Could you check a few things on this model? Use its own coordinates, in mm. A direction names the side the tool comes from. Round coordinates to 2 decimals unless told otherwise and drop trailing zeros. Order: outer loops, then holes, each group sorted by start corner. A loop starts at its lowest first (then second) coordinate and runs counter-clockwise, first axis right, second up.
Solid Edge part; units mm, degrees
sketch "Sketch1" plane through (0, 0, 0) normal (0, 0, 1) x (1, 0, 0)
  circle A0 centre (0, 0) radius 10.5
extrude "Protrusion1" add sketch "Sketch1" along normal blind 2
sketch "Sketch2" plane through (0, 0, 2) normal (0, 0, 1) x (1, 0, 0)
  line L0 (-3.25, -3.25) -> (3.25, -3.25)
  line L1 (3.25, -3.25) -> (3.25, 3.25)
  line L2 (3.25, 3.25) -> (-3.25, 3.25)
  line L3 (-3.25, 3.25) -> (-3.25, -3.25)
extrude "Extrusionsausprägung_2" add sketch "Sketch2" along normal blind 6.5
chamfer "Fase_1" distance 1 angle 45 1 edges at (-10.5, 0, 2)
hole "Bohrung_1" at (0, 0, 0) direction (0, 0, 1) diameter 4 end through all
Q1. Imagine slicing it at A-A, the plane x = 0. Please give me the cut outline in (y, z).
Q2. Imagine slicing it at C-C, the plane z = 1.5. Please give me the cut outline in (x, y).
Q3. We'd pull the mould along X, two halves only. Please class faces 4 (the cylindrical face through (-2, 0, 4)), 5 (the flat face through (0, 3.25, 5)), 6 (the flat face through (-3.25, 0, 5)): released by +X, released by -X, zero draft, split by the parting line, or undercut.
Q4. For faces 1 (the flat face through (2.2, 0.1, 0)), 2 (the flat face through (3.25, 0, 5)), 3 (the flat face through (0, -3.25, 5)), which set-ups out of +Z, -Z, +X, -X, +Y, -Y let a thin tool reach every point of the face, with its end or its side?
Q5. Imagine slicing it at D-D, the plane z = 2.75. Please give me the cut outline in (x, y), then the cut area to 3 significant figures.
Q6. I need wall thicknesses on L1, parallel to X at y = 0, z = 4; L2, parallel to Z at x = -4, y = 5. Which ranges of each line are inside material? Lowest first, please.
Q7. For P1, Ø5, axis at x = -0.5, z = 6, coming from the -Y side; P2, Ø5, axis at x = 6, z = 1, coming from the +Y side; P3, Ø3, axis at y = -4, z = 2, coming from the -X side, each with a flat end and sliding along its axis, tell me the tip position at first contact or that it passes through.
Filled in:
1. outline: (-10.5, 0) - (-2, 0) - (-2, 8.5) - (-3.25, 8.5) - (-3.25, 2) - (-9.5, 2) - (-10.5, 1) - close; (2, 0) - (10.5, 0) - (10.5, 1) - (9.5, 2) - (3.25, 2) - (3.25, 8.5) - (2, 8.5) - close
2. outline: circle Ø20 at (0, 0); hole circle Ø4 at (0, 0)
3. face 4: undercut
3. face 5: zero draft
3. face 6: released by -X
4. face 1: -Z, +X, -X, +Y, -Y
4. face 2: +Z, +X, +Y, -Y
4. face 3: +Z, +X, -X, -Y
5. outline: (-3.25, -3.25) - (3.25, -3.25) - (3.25, 3.25) - (-3.25, 3.25) - close; hole circle Ø4 at (0, 0)
5. area: 29.7 mm2
6. L1: x = -3.25 to -2, 2 to 3.25
6. L2: z = 0 to 2
7. P1: stops at y = -3.25
7. P2: stops at y = 9.9
7. P3: stops at x = -10.1
